For this review, use the dimensioned drawing (mm, ordinates from the lowest corner) and the shaded views. A direction names the side the tool comes from. Give positions to 0.01 mm unless a question says otherwise; leave off trailing zeros. Loops run counter-clockwise (first coordinate to the right, second up) from the corner with the lowest first, then second, coordinate; pieces in that order, holes last. Notation, with made-up numbers: (63.25, 36.25) - (109.25, 36.25) arc R21 ccw to (109.25, 72.25) - close; hole circle Ø9 at (11.5, 54.5). An arc over 180 degrees is marked (long way). Write each question's results on one line, items separated by ' | '.
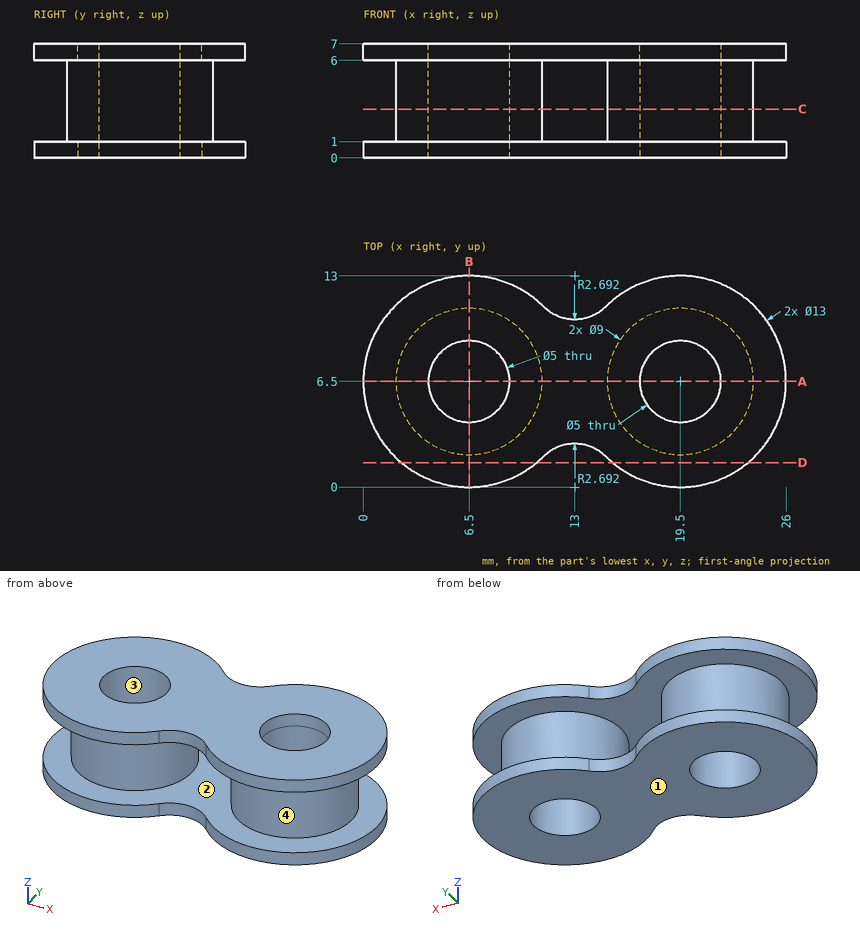
Item 1: Clearance check with flat-ended pins moving along their axes: P1, Ø2, axis at y = 5.5, z = 2.5, coming from the +X side; P2, Ø1, axis at x = 19, y = 7, coming from the +Z side; P3, Ø1, axis at y = 9.5, z = 4, coming from the +X side. State where each tip first meets the part, or that it passes through.
Output values:
P1: stops at x = 24 | P2: passes through | P3: stops at x = 23.24
Item 2: We need section B-B on x = 6.5. Give the boundary of the cut face in (y, z).
Output values:
outline: (0, 0) - (4, 0) - (4, 7) - (0, 7) - (0, 6) - (2, 6) - (2, 1) - (0, 1) - close; (9, 0) - (13, 0) - (13, 1) - (11, 1) - (11, 6) - (13, 6) - (13, 7) - (9, 7) - close
Item 3: Draft analysis for pull direction X (two halves, no side actions). For the marked faces 1 and 2, state which applies: +X half, -X half, draft (parallel to the pull), parting line (faces both ways), or undercut.
Output values:
face 1: draft | face 2: undercut
Item 4: We need section D-D on y = 1.5. Give the boundary of the cut face in (x, z).
Output values:
outline: (2.35, 0) - (10.65, 0) - (10.65, 1) - (2.35, 1) - close; (2.35, 6) - (10.65, 6) - (10.65, 7) - (2.35, 7) - close; (15.35, 0) - (23.65, 0) - (23.65, 1) - (15.35, 1) - close; (15.35, 6) - (23.65, 6) - (23.65, 7) - (15.35, 7) - close
Item 5: Wall thickness on probe 1 along Y at (x, z) = (19.5, 3.9); probe 2 along Z at (x, y) = (3.5, 3); probe 3 along Y at (x, z) = (19.5, 6.6): over which ranges is each line inside the solid? List them lowest first.
Output values:
probe 1: y = 2 to 4, 9 to 11 | probe 2: z = 0 to 1, 6 to 7 | probe 3: y = 0 to 4, 9 to 13
Item 6: Tool access review of the marked faces 3 and 4: name each direction out of +Z, -Z, +X, -X, +Y, -Y from which nothing blocks a thin tool from reaching the whole face with its end or side.
Output values:
face 3: +Z, -Z | face 4: none
Item 7: We need section A-A on y = 6.5. Give the boundary of the cut face in (x, z).
Output values:
outline: (0, 0) - (4, 0) - (4, 7) - (0, 7) - (0, 6) - (2, 6) - (2, 1) - (0, 1) - close; (9, 0) - (17, 0) - (17, 7) - (9, 7) - close; (22, 0) - (26, 0) - (26, 1) - (24, 1) - (24, 6) - (26, 6) - (26, 7) - (22, 7) - close; hole (11, 1) - (15, 1) - (15, 6) - (11, 6) - close
Item 8: We need section C-C on z = 3. Give the boundary of the cut face in (x, y).
Output values:
outline: circle Ø9 at (6.5, 6.5); circle Ø9 at (19.5, 6.5); hole circle Ø5 at (6.5, 6.5); hole circle Ø5 at (19.5, 6.5)
